from build123d import *

# Parameters (mm, degrees)
F0_W     = 76.2
F0_H     = 101.6
F1_DEPTH = 12.7
F2_R     = 12.7


with BuildPart() as f1:
    # F0 (on Top) → F1 (new body, symmetric)
    with BuildSketch(Plane.XY):
        Rectangle(F0_W, F0_H)
    extrude(amount=F1_DEPTH, both=True)

    # F2
    f2_edges = [f1.edges().sort_by_distance(p)[0] for p in [
        (0, -50.8, 12.7),
        (38.1, 0, 12.7),
        (-38.1, 0, 12.7),
        (0, 50.8, 12.7),
    ]]
    fillet(f2_edges, radius=F2_R)


solid = f1.part
Verification items for the finished model (mm, model axes). Give positions to 0.01 mm unless a question says otherwise; leave off trailing zeros. Order: outer loops, then holes, each group sorted by start corner. A loop starts at its lowest first (then second) coordinate and runs counter-clockwise, first axis right, second up. Notation, with made-up numbers: M -17.5,-19.75 L -11.5,-19.75 A34 ccw -11.5,16.25 Z; hole C 17,-0.5 d3. An arc over 180 degrees is marked long. Answer as a JSON object with one key per item and string values. Group by question number.
1) Cross-section at D-D (z = 4.75). Enter the section's corners in (x, y), then the cut area to 3 significant figures.
2) Depth check by flat-ended pin: pin 1 Ø5 at (y, z) = (12, 7.5) entering from +X; pin 2 Ø1 at (x, z) = (4, 7.5) entering from -Y; pin 3 Ø1.5 at (y, z) = (-16, 2.5) entering from -X. Enter the tip coordinate at first touch or a pass-through.
3) Cross-section at A-A (x = 9). Enter the section's corners in (y, z).
4) Scan lines: line 1 along X through (y, z) = (34.5, 0.5); line 2 along Y through (x, z) = (29.5, 5); line 3 along X through (y, z) = (12, 11). Record each from-to range of solid material in increasing order. Write a range as [from, to].
5) Cross-section at B-B (y = -35). Enter the section's corners in (x, z), then the cut area to 3 significant figures.
6) Cross-section at C-C (z = 10.5). Enter the section's corners in (x, y), then the cut area to 3 significant figures.
Result sheet:
{
 "1": {"outline": "M -37.18,-49.88 L 37.18,-49.88 L 37.18,49.88 L -37.18,49.88 Z", "area": "7,420 mm2"},
 "2": {"pin 1": "stops at x = 37.07", "pin 2": "stops at y = -48.7", "pin 3": "stops at x = -37.98"},
 "3": {"outline": "M -50.8,-12.7 L 50.8,-12.7 L 50.8,0 A12.7 ccw 38.1,12.7 L -38.1,12.7 A12.7 ccw -50.8,0 Z"},
 "4": {"line 1": "x = [-38.09, 38.09]", "line 2": "y = [-49.77, 49.77]", "line 3": "x = [-31.75, 31.75]"},
 "5": {"outline": "M -38.1,-12.7 L 38.1,-12.7 L 38.1,0 A12.7 ccw 25.4,12.7 L -25.4,12.7 A12.7 ccw -38.1,0 Z", "area": "1,870 mm2"},
 "6": {"outline": "M -32.54,-45.24 L 32.54,-45.24 L 32.54,45.24 L -32.54,45.24 Z", "area": "5,890 mm2"}
}
